Can you work these out from the model? Positions are in its coordinate system, mm. Face numbers are marked on the shaded views. A direction names the side the tool comes from. Round coordinates to 2 decimals unless told otherwise and drop trailing zeros. Loops run counter-clockwise (first coordinate to the right, second up) from the corner with the lowest first, then second, coordinate; pieces in that order, holes last.
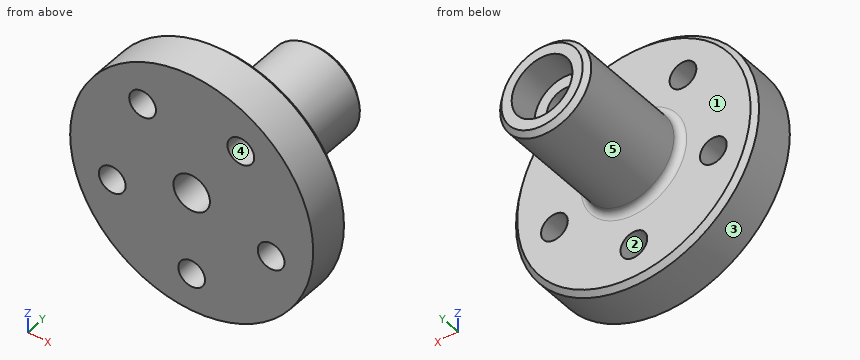
from build123d import *

# Parameters (mm, degrees)
SKETCH1_R           = 50.8
BOSS_EXTRUDE1_DEPTH = 19.05
CHAMFER1_SIZE       = 2.032
SKETCH2_R           = 5.588
CUT_EXTRUDE2_DEPTH  = 75.324844433
SKETCH4_R           = 19.05
BOSS_EXTRUDE2_DEPTH = 50.8
FILLET1_R           = 3.048
CHAMFER2_SIZE       = 2.032
SKETCH5_R           = 12.7
CUT_EXTRUDE3_DEPTH  = 12.7
SKETCH6_R           = 7.62
CUT_EXTRUDE4_DEPTH  = 92.800885072


with BuildPart() as part:
    # Sketch1 → Boss-Extrude1 (new body)
    with BuildSketch(Plane(origin=(0, 0, 0), x_dir=(1, 0, 0), z_dir=(0, 1, 0))):
        with Locations(Location((0, 0, 0), (0, 0, 90))):
            Circle(SKETCH1_R)
    extrude(amount=BOSS_EXTRUDE1_DEPTH)

    # Chamfer1
    chamfer1_edges = [part.edges().sort_by_distance(p)[0] for p in [
        (0, 19.05, 50.8),
    ]]
    chamfer(chamfer1_edges, length=CHAMFER1_SIZE)

    # Sketch2 → Cut-Extrude2 (cut, through all)
    with BuildSketch(Plane(origin=(0, 19.05, 0), x_dir=(1, 0, 0), z_dir=(0, 1, 0))):
        with Locations(Location((0, 34.925, 0), (0, 0, 270))):
            Circle(SKETCH2_R)
        with Locations(Location((33.215648832, 10.792418529, 0), (0, 0, 270))):
            Circle(SKETCH2_R)
        with Locations(Location((20.528399936, -28.254918529, 0), (0, 0, 270))):
            Circle(SKETCH2_R)
        with Locations(Location((-20.528399936, -28.254918529, 0), (0, 0, 270))):
            Circle(SKETCH2_R)
        with Locations(Location((-33.215648832, 10.792418529, 0), (0, 0, 270))):
            Circle(SKETCH2_R)
    extrude(amount=-CUT_EXTRUDE2_DEPTH, mode=Mode.SUBTRACT)

    # Sketch4 → Boss-Extrude2 (add)
    with BuildSketch(Plane(origin=(0, 19.05, 0), x_dir=(1, 0, 0), z_dir=(0, 1, 0))):
        with Locations(Location((0, 0, 0), (0, 0, 270))):
            Circle(SKETCH4_R)
    extrude(amount=BOSS_EXTRUDE2_DEPTH)

    # Fillet1
    fillet1_edges = [part.edges().sort_by_distance(p)[0] for p in [
        (0, 19.05, -19.05),
    ]]
    fillet(fillet1_edges, radius=FILLET1_R)

    # Chamfer2
    chamfer2_edges = [part.edges().sort_by_distance(p)[0] for p in [
        (0, 69.85, -19.05),
    ]]
    chamfer(chamfer2_edges, length=CHAMFER2_SIZE)

    # Sketch5 → Cut-Extrude3 (cut)
    with BuildSketch(Plane(origin=(0, 69.85, 0), x_dir=(1, 0, 0), z_dir=(0, 1, 0))):
        with Locations(Location((0, 0, 0), (0, 0, 270))):
            Circle(SKETCH5_R)
    extrude(amount=-CUT_EXTRUDE3_DEPTH, mode=Mode.SUBTRACT)

    # Sketch6 → Cut-Extrude4 (cut, through all)
    with BuildSketch(Plane(origin=(0, 57.15, 0), x_dir=(1, 0, 0), z_dir=(0, 1, 0))):
        with Locations(Location((0, 0, 0), (0, 0, 270))):
            Circle(SKETCH6_R)
    extrude(amount=-CUT_EXTRUDE4_DEPTH, mode=Mode.SUBTRACT)


solid = part.part
(1) If we section it at C-C, the plane y = 13: List the corners of the cut face in (x, z) for me (3 decimals), then the cut area to 3 significant figures.
Worked answers:
outline: circle Ø101.6 at (0, 0); hole circle Ø11.176 at (-33.216, -10.792); hole circle Ø11.176 at (-20.528, 28.255); hole circle Ø15.24 at (0, 0); hole circle Ø11.176 at (0, -34.925); hole circle Ø11.176 at (20.528, 28.255); hole circle Ø11.176 at (33.216, -10.792)
area: 7,430 mm2
(2) For the marked faces 4 and 5, which set-ups out of +Z, -Z, +X, -X, +Y, -Y let a thin tool reach every point of the face, with its end or its side?
Worked answers:
face 4: +Y, -Y
face 5: +Y
(3) If we section it at D-D, the plane y = 52.5: List the corners of the cut face in (x, z) for me, then the cut area to 3 significant figures.
Worked answers:
outline: circle Ø38.1 at (0, 0); hole circle Ø15.24 at (0, 0)
area: 958 mm2
(4) If I drill on line 1 (X direction, y = 22, z = 1.5); line 2 (Y direction, x = 26.5, z = -24.5); line 3 (Z direction, x = 5, y = 60), over which ranges is the centre line in solid material (lowest first)?
Worked answers:
line 1: x = -18.99 to -7.47, 7.47 to 18.99
line 2: y = 0 to 19.05
line 3: z = -18.38 to -11.67, 11.67 to 18.38
(5) If we section it at B-B, the plane z = 0: List the corners of the cut face in (x, y) for me, then the cut area to 3 significant figures.
Worked answers:
outline: (-50.8, 0) - (-7.62, 0) - (-7.62, 57.15) - (-12.7, 57.15) - (-12.7, 69.85) - (-17.02, 69.85) - (-19.05, 67.82) - (-19.05, 22.1) arc R3.05 cw to (-22.1, 19.05) - (-48.77, 19.05) - (-50.8, 17.02) - close; (7.62, 0) - (50.8, 0) - (50.8, 17.02) - (48.77, 19.05) - (22.1, 19.05) arc R3.05 cw to (19.05, 22.1) - (19.05, 67.82) - (17.02, 69.85) - (12.7, 69.85) - (12.7, 57.15) - (7.62, 57.15) - close
area: 2,670 mm2
(6) Will these pins go through, and if not, where does the flat tip stop? P1, Ø12, axis at x = 23.5, y = 21, coming from the +Z side; P2, Ø14.5, axis at x = 0, z = -34.925, coming from the -Y side; P3, Ø4, axis at x = -31.5, y = 16.5, coming from the -Z side; P4, Ø12, axis at y = 23, z = -39, coming from the -X side.
Worked answers:
P1: stops at z = 47.11
P2: stops at y = 0
P3: stops at z = -41.36
P4: stops at x = -34.77
(7) If we mould it in two halves opening along Z, with no side actions, what happens to the marked faces 1, 2 and 3? For each: released by +Z, released by -Z, zero draft, split by the parting line, or undercut.
Worked answers:
face 1: zero draft
face 2: undercut
face 3: split by the parting line
(8) If we section it at A-A, the plane x = 0: List the corners of the cut face in (y, z) for me, then the cut area to 3 significant figures.
Worked answers:
outline: (0, -50.8) - (17.02, -50.8) - (19.05, -48.77) - (19.05, -40.51) - (0, -40.51) - close; (0, -29.34) - (19.05, -29.34) - (19.05, -22.1) arc R3.05 cw to (22.1, -19.05) - (67.82, -19.05) - (69.85, -17.02) - (69.85, -12.7) - (57.15, -12.7) - (57.15, -7.62) - (0, -7.62) - close; (0, 7.62) - (57.15, 7.62) - (57.15, 12.7) - (69.85, 12.7) - (69.85, 17.02) - (67.82, 19.05) - (22.1, 19.05) arc R3.05 cw to (19.05, 22.1) - (19.05, 48.77) - (17.02, 50.8) - (0, 50.8) - close
area: 2,460 mm2
